Verification items for the finished model (mm, model axes). Give positions to 0.01 mm unless a question says otherwise; leave off trailing zeros. Order: outer loops, then holes, each group sorted by start corner. A loop starts at its lowest first (then second) coordinate and runs counter-clockwise, first axis right, second up. Notation, with made-up numbers: (-7, 39) -> (2, 39) arc R24 ccw to (2, 69) -> close; hole circle Ø4 at (53.5, 13.25). An arc over 180 degrees is marked (long way). Return JSON: item names as keys, results as strings. Group by question number.
(1) Cross-section at C-C on z = 54.5. Enter the section's corners in (x, y), then the cut area to 3 significant figures.
(2) Cross-section at B-B on y = 0. Enter the section's corners in (x, z).
(3) Release check for a two-part mould opening along Z. For faces 1 (the face through (0, 0, 60)), 2 (the face through (-4.291, 0, 20)), 3 (the face through (0, 0, 0)) record: pulls with the +Z half, pulls with the -Z half, needs draft (parallel to the pull), parting line crosses it, or undercut.
(4) Cross-section at A-A on x = 0. Enter the section's corners in (y, z).
(5) Thickness scan on line 1 along Z through (x, y) = (-2, -16); line 2 along X through (y, z) = (-7, 38.5); line 3 along Y through (x, z) = (0.5, 29) (3 decimals). Record the ranges inside material, lowest first.
(6) Cross-section at D-D on x = 14. State how many separate pieces and enclosed holes the cut face has, then the cut area to 3 significant figures.
(7) Depth check by flat-ended pin: pin 1 Ø4.5 at (y, z) = (-0.5, 43.5) entering from +X; pin 2 Ø1 at (y, z) = (18.5, 31.5) entering from +X; pin 3 Ø12 at (x, z) = (19.5, 50.5) entering from +Y; pin 4 Ø1.8 at (y, z) = (-0.5, 18.5) entering from +X. Enter the tip coordinate at first touch or a pass-through.
from build123d import *

# Parameters (mm, degrees)
F0_R      = 25
F1_DEPTH  = 60
F2_W      = 61.5676790476
F2_H      = 184.1998919845
F3_DEPTH  = 6
F10_SIZE  = 1
F11_SIZE  = 1
F12_DEPTH = 2


with BuildPart() as f1:
    # F0 (on Top) → F1 (new body)
    with BuildSketch(Plane.XY):
        Circle(F0_R)
    extrude(amount=F1_DEPTH)


with BuildPart() as f3:
    # F2 (on Top) → F3 (new body)
    with BuildSketch(Plane.XY):
        with Locations((-161.507062614, 31.8613536656)):
            Rectangle(F2_W, F2_H)
    extrude(amount=F3_DEPTH)


with BuildPart() as f4_1:
    # F4: copy of F3
    add(f3.part.moved(Location((188, 0, 17))))


with BuildPart() as f5_1:
    # F5: copy of F4_1
    add(f4_1.part.moved(Location((0, 0, 17))))


with BuildPart() as f7_1:
    # F7: copy of F4_1
    add(f4_1.part.moved(Location((0, 0, 23))))


with BuildPart() as f1_1:
    add(f1.part)

    # F8: cut F4_1, F7_1
    add(f4_1.part, mode=Mode.SUBTRACT)
    add(f7_1.part, mode=Mode.SUBTRACT)

    # F10
    f10_edges = [f1_1.edges().sort_by_distance(p)[0] for p in [
        (-25, 0, 60),
    ]]
    chamfer(f10_edges, length=F10_SIZE)

    # F11
    f11_edges = [f1_1.edges().sort_by_distance(p)[0] for p in [
        (-25, 0, 0),
    ]]
    chamfer(f11_edges, length=F11_SIZE)

    # F12 (add): a face of the model
    f12_faces = [f1_1.faces().sort_by_distance(p)[0] for p in [
        (8.3329049889, 0, 40),
    ]]
    extrude(f12_faces, amount=F12_DEPTH)


solid = f1_1.part
Verdict:
{
 "1": {"outline": "circle Ø50 at (0, 0)", "area": "1,960 mm²"},
 "2": {"outline": "(-25, 1) -> (-24, 0) -> (24, 0) -> (25, 1) -> (25, 17) -> (-4.29, 17) -> (-4.29, 23) -> (25, 23) -> (25, 42) -> (-4.29, 42) -> (-4.29, 46) -> (25, 46) -> (25, 59) -> (24, 60) -> (-24, 60) -> (-25, 59) -> close"},
 "3": {"face 1": "pulls with the +Z half", "face 2": "undercut", "face 3": "pulls with the -Z half"},
 "4": {"outline": "(-25, 1) -> (-24, 0) -> (24, 0) -> (25, 1) -> (25, 17) -> (-25, 17) -> close; (-25, 23) -> (25, 23) -> (25, 42) -> (-25, 42) -> close; (-25, 46) -> (25, 46) -> (25, 59) -> (24, 60) -> (-24, 60) -> (-25, 59) -> close"},
 "5": {"line 1": "0 to 17, 23 to 42, 46 to 60", "line 2": "-24 to 24", "line 3": "-24.995 to 24.995"},
 "6": {"separate pieces": "3", "enclosed holes": "0", "area": "2,070 mm²"},
 "7": {"pin 1": "x = 25", "pin 2": "x = 17.35", "pin 3": "y = 21.04", "pin 4": "x = -4.29"}
}
